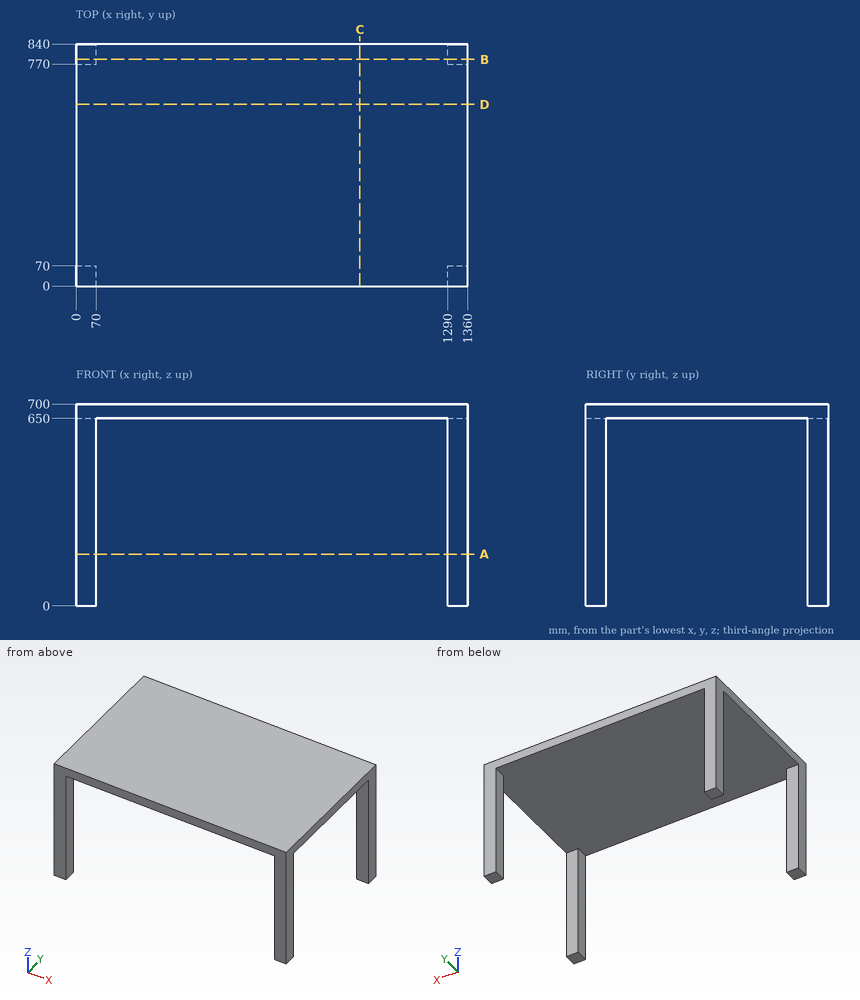
Input: dimensioned drawing with shaded views. Units: mm. Origin: part minimum x, y, z. Coordinates: 2 decimals unless noted, no trailing zeros. Write each loop counter-clockwise with the first axis right and the second up, starting at its lowest first coordinate (ties: lowest second). Pieces come first, ordered by that corner, then holes. Notation, with made-up numbers: M -37.75,17 L -3.75,17 A20 ccw -3.75,30 Z; hole C -20,40.25 d9. An arc over 180 degrees is marked long. Answer as a JSON object with one key per item and string values. Group by question number.
(1) Section C-C on x = 985. Output: boundary loops of the cut face in (y, z).
(2) Ray query, line 1 along X through (y, z) = (791, 566); line 2 along Z through (x, y) = (1236, 221.5). Return the intervals inside material, ascending. Write a range as [from, to].
(3) Contact query for a flat-ended pin moving along its axis: P1, Ø4, axis at x = 1092, y = 96.5, coming from the -Z side. Output: stop coordinate, or through.
(4) Section B-B on y = 787. Output: boundary loops of the cut face in (x, z).
(5) Section D-D on y = 630.5. Output: boundary loops of the cut face in (x, z).
(6) Section A-A on z = 179. Output: boundary loops of the cut face in (x, y).
Result set:
{
 "1": {"outline": "M 0,650 L 840,650 L 840,700 L 0,700 Z"},
 "2": {"line 1": "x = [0, 70], [1290, 1360]", "line 2": "z = [650, 700]"},
 "3": {"P1": "stops at z = 650"},
 "4": {"outline": "M 0,0 L 70,0 L 70,650 L 1290,650 L 1290,0 L 1360,0 L 1360,700 L 0,700 Z"},
 "5": {"outline": "M 0,650 L 1360,650 L 1360,700 L 0,700 Z"},
 "6": {"outline": "M 0,0 L 70,0 L 70,70 L 0,70 Z; M 0,770 L 70,770 L 70,840 L 0,840 Z; M 1290,0 L 1360,0 L 1360,70 L 1290,70 Z; M 1290,770 L 1360,770 L 1360,840 L 1290,840 Z"}
}
